Geometry check sheet. Reference: drawing and pictorial views, mm from the part's lowest x, y, z. A direction names the side the tool comes from. Give positions to 0.01 mm unless a question says otherwise; leave off trailing zeros. Loops run counter-clockwise (first coordinate to the right, second up) from the corner with the lowest first, then second, coordinate; pieces in that order, holes last. Notation, with made-up numbers: (68, -5.75) - (100, -5.75) arc R10 cw to (100, 2.25) - close; hole circle Ø11 at (-25.75, 74). An arc over 180 degrees is marked (long way). Answer in a Markdown table with one row per item. Add a question column.
(1) Sectioned sample at A-A on y = 6.5. Enter the section's corners in (x, z), then the cut area to 3 significant figures.
(2) Thickness scan on L1, parallel to Y at x = 6.5, z = 3.4; L2, parallel to X at y = 4, z = 3.3; L3, parallel to X at y = 7.25, z = 0.35. Record the ranges inside material, lowest first.
(3) Sectioned sample at C-C on z = 1.8. Enter the section's corners in (x, y).
(4) Set-up check for the marked faces 1 and 2: record each of +Z, -Z, +X, -X, +Y, -Y from which the full face is reachable in a straight line by a thin tool's end or side.
(5) Sectioned sample at D-D on x = 2.75. Enter the section's corners in (y, z).
(6) Draft check along X on the marked faces 3, 4 and 5. Enter one of: released by +X, released by -X, zero draft, split by the parting line, or undercut.
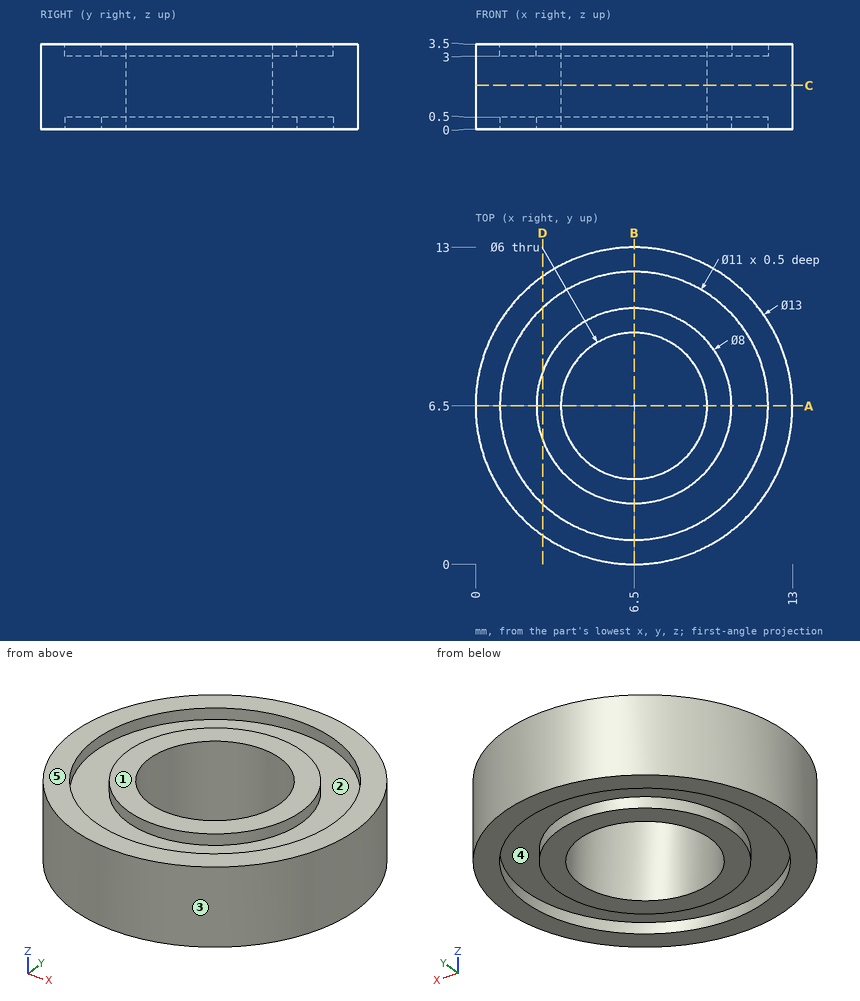
Reply:
| question | item | result |
|---|---|---|
| 1 | outline | (0, 0) - (1, 0) - (1, 0.5) - (2.5, 0.5) - (2.5, 0) - (3.5, 0) - (3.5, 3.5) - (2.5, 3.5) - (2.5, 3) - (1, 3) - (1, 3.5) - (0, 3.5) - close; (9.5, 0) - (10.5, 0) - (10.5, 0.5) - (12, 0.5) - (12, 0) - (13, 0) - (13, 3.5) - (12, 3.5) - (12, 3) - (10.5, 3) - (10.5, 3.5) - (9.5, 3.5) - close |
| 1 | area | 21.5 mm^2 |
| 2 | L1 | 0 to 1, 2.5 to 3.5, 9.5 to 10.5, 12 to 13 |
| 2 | L2 | 0.5 to 1.6, 3.38 to 4.84, 8.16 to 9.62, 11.4 to 12.5 |
| 2 | L3 | 0.04 to 1.05, 2.57 to 3.6, 9.4 to 10.43, 11.95 to 12.96 |
| 3 | outline | circle Ø13 at (6.5, 6.5); hole circle Ø6 at (6.5, 6.5) |
| 4 | face 1 | +Z, +X, -X, +Y, -Y |
| 4 | face 2 | +Z |
| 5 | outline | (1.19, 0) - (2.48, 0) - (2.48, 0.5) - (5.11, 0.5) - (5.11, 0) - (7.89, 0) - (7.89, 0.5) - (10.52, 0.5) - (10.52, 0) - (11.81, 0) - (11.81, 3.5) - (10.52, 3.5) - (10.52, 3) - (7.89, 3) - (7.89, 3.5) - (5.11, 3.5) - (5.11, 3) - (2.48, 3) - (2.48, 3.5) - (1.19, 3.5) - close |
| 6 | face 3 | split by the parting line |
| 6 | face 4 | undercut |
| 6 | face 5 | zero draft |
